Part model, mm, in its own coordinate system. Face numbers are marked on the shaded views. A direction names the side the tool comes from. Coordinates: 2 decimals unless noted, no trailing zeros. Order: outer loops, then holes, each group sorted by start corner. A loop starts at its lowest first (then second) coordinate and runs counter-clockwise, first axis right, second up.
from build123d import *

# Parameters (mm, degrees)
SKETCH_1_W           = 20
SKETCH_1_H           = 10
EXTRUDE_1_DEPTH      = 5
SKETCH_2_W           = 20
SKETCH_2_H           = 2.5
EXTRUDE_2_DEPTH      = 15
EXTRUDE_3_DEPTH      = 12.5
EXTRUDE_3_DEPTH_BACK = 7.5
SKETCH_3_R           = 0.75


with BuildPart() as part:
    # Sketch 1 → Extrude 1 (new body)
    with BuildSketch(Plane.XY):
        with Locations((10, 5)):
            Rectangle(SKETCH_1_W, SKETCH_1_H)
    extrude(amount=EXTRUDE_1_DEPTH)

    # Sketch 2 → Extrude 2 (add)
    with BuildSketch(Plane.XY.offset(5)):
        with Locations((10, 1.25)):
            Rectangle(SKETCH_2_W, SKETCH_2_H)
    extrude(amount=EXTRUDE_2_DEPTH)

    # Sketch 3 → Extrude 3 (add, two sides: drawn at the far end of the back side and taken through both)
    with BuildSketch(Plane.XY.offset(5).offset(-EXTRUDE_3_DEPTH_BACK)):
        with Locations(Location((12.5, 6.25, 0), (0, 0, 180))):
            Circle(SKETCH_3_R)
        with Locations(Location((17.5, 6.25, 0), (0, 0, 180))):
            Circle(SKETCH_3_R)
        with Locations(Location((2.5, 6.25, 0), (0, 0, 180))):
            Circle(SKETCH_3_R)
        with Locations(Location((7.5, 6.25, 0), (0, 0, 180))):
            Circle(SKETCH_3_R)
    extrude(amount=EXTRUDE_3_DEPTH + EXTRUDE_3_DEPTH_BACK)


solid = part.part
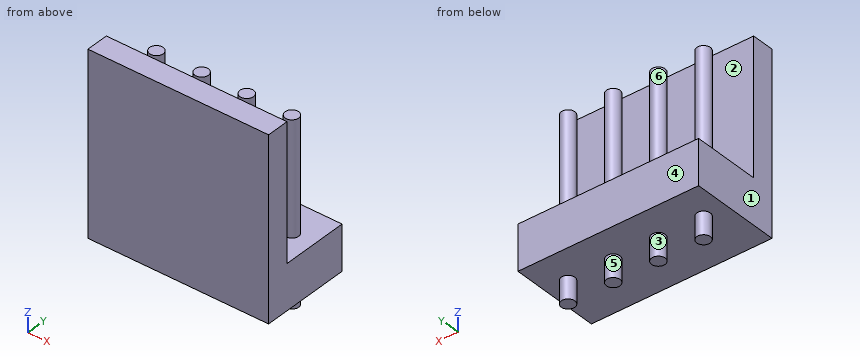
Q1. Wall check: line 1 along Y through (x, z) = (2.5, 7.75); line 2 along X through (y, z) = (6, 16.5); line 3 along Z through (x, y) = (7.5, 1.25). Give the ranges that are in metal, low to high.
Results list:
line 1: y = 0 to 2.5, 5.5 to 7
line 2: x = 1.79 to 3.21, 6.79 to 8.21, 11.79 to 13.21, 16.79 to 18.21
line 3: z = 0 to 20
Q2. Cut at A-A on z = 13.25. Write the cut outline in (x, y).
Results list:
outline: (0, 0) - (20, 0) - (20, 2.5) - (0, 2.5) - close; circle Ø1.5 at (2.5, 6.25); circle Ø1.5 at (7.5, 6.25); circle Ø1.5 at (12.5, 6.25); circle Ø1.5 at (17.5, 6.25)
Q3. Cut at C-C on z = -0.5. Write the cut outline in (x, y), and give its area (3 significant figures).
Results list:
outline: circle Ø1.5 at (2.5, 6.25); circle Ø1.5 at (7.5, 6.25); circle Ø1.5 at (12.5, 6.25); circle Ø1.5 at (17.5, 6.25)
area: 7.07 mm2
Q4. Pin check, flat tips, straight feed: pin 1 Ø1.6 at (x, y) = (17.5, 6) entering from +Z; pin 2 Ø4.5 at (x, z) = (7, 15.5) entering from +Y; pin 3 Ø6 at (x, y) = (10, 3) entering from +Z. Stop position of each tip, or through.
Results list:
pin 1: stops at z = 17.5
pin 2: stops at y = 7
pin 3: stops at z = 20
Q5. Mould opens along Y. For the marked faces 1, 2 and 3 say: pulls with the +Y half, pulls with the -Y half, needs draft (parallel to the pull), parting line crosses it, or undercut.
Results list:
face 1: needs draft
face 2: undercut
face 3: parting line crosses it
Q6. Cut at D-D on y = 1. Write the cut outline in (x, z).
Results list:
outline: (0, 0) - (20, 0) - (20, 20) - (0, 20) - close
Q7. Which spindle directions (+Z, -Z, +X, -X, +Y, -Y) get a long thin tool onto all of the face, cutting with end or side? Do the marked faces 4, 5 and 6. Say none if no direction does.
Results list:
face 4: +Z, -Z, +X, -X, +Y
face 5: -Z
face 6: +Z
Q8. Cut at B-B on x = 12.5. Write the cut outline in (y, z), and give its area (3 significant figures).
Results list:
outline: (0, 0) - (5.5, 0) - (5.5, -2.5) - (7, -2.5) - (7, 0) - (10, 0) - (10, 5) - (7, 5) - (7, 17.5) - (5.5, 17.5) - (5.5, 5) - (2.5, 5) - (2.5, 20) - (0, 20) - close
area: 110 mm2
